Check sheet for the modelled part. Datum: model origin and axes. Units: mm. Face numbers are marked on the shaded views. Round coordinates to 2 decimals unless told otherwise and drop trailing zeros. Order: outer loops, then holes, each group sorted by start corner. A loop starts at its lowest first (then second) coordinate and runs counter-clockwise, first axis right, second up. Notation, with made-up numbers: (18, 80) -> (75, 80) arc R7 ccw to (75, 88) -> close; hole circle Ø8 at (33.5, 16). An arc over 180 degrees is marked (long way). Answer in a Markdown table with one row per item.
```python
from build123d import *

# Parameters (mm, degrees)
SKETCH1_W          = 76.2
SKETCH1_H          = 182.7422304
BASE_FLANGE1_DEPTH = 1.5875
CUT_EXTRUDE1_REACH = 199.999
SKETCH6_R          = 3.3782
SKETCH7_R          = 9.525
CUT_EXTRUDE2_DEPTH = 198.999199311
HEM1_START         = -182.7422304
HEM1_DEPTH         = 182.7422304
HEM1_2_DEPTH       = 182.7422304


# Read off the part's stored shape, not the designer's step: Hem1
# Sheet-metal steps are written as plain solids
with BuildPart() as part:
    # Sketch1 → Base-Flange1 (new body)
    with BuildSketch(Plane(origin=(0, 0, 0), x_dir=(1, 0, 0), z_dir=(0, 1, 0))):
        with Locations((-38.1, 91.3711152)):
            Rectangle(SKETCH1_W, SKETCH1_H)
    extrude(amount=-BASE_FLANGE1_DEPTH)

    # Sketch6 → Cut-Extrude1 (cut, up to next)
    with BuildSketch(Plane(origin=(0, 0, 0), x_dir=(1, 0, 0), z_dir=(0, 1, 0)), mode=Mode.PRIVATE) as cut_extrude1_sk1:
        with Locations(Location((-57.15, 170.0422304, 0), (0, 0, 270))):
            Circle(SKETCH6_R)
    cut_extrude1_tool1 = extrude(cut_extrude1_sk1.sketch, amount=-CUT_EXTRUDE1_REACH, mode=Mode.PRIVATE) & part.part
    # Sketch6 → Cut-Extrude1 (cut, up to next)
    with BuildSketch(Plane(origin=(0, 0, 0), x_dir=(1, 0, 0), z_dir=(0, 1, 0)), mode=Mode.PRIVATE) as cut_extrude1_sk2:
        with Locations(Location((-19.05, 170.0422304, 0), (0, 0, 270))):
            Circle(SKETCH6_R)
    cut_extrude1_tool2 = extrude(cut_extrude1_sk2.sketch, amount=-CUT_EXTRUDE1_REACH, mode=Mode.PRIVATE) & part.part
    # Sketch6 → Cut-Extrude1 (cut, up to next)
    with BuildSketch(Plane(origin=(0, 0, 0), x_dir=(1, 0, 0), z_dir=(0, 1, 0)), mode=Mode.PRIVATE) as cut_extrude1_sk3:
        with Locations(Location((-19.05, 107.14228, 0), (0, 0, 270))):
            Circle(SKETCH6_R)
    cut_extrude1_tool3 = extrude(cut_extrude1_sk3.sketch, amount=-CUT_EXTRUDE1_REACH, mode=Mode.PRIVATE) & part.part
    # Sketch6 → Cut-Extrude1 (cut, up to next)
    with BuildSketch(Plane(origin=(0, 0, 0), x_dir=(1, 0, 0), z_dir=(0, 1, 0)), mode=Mode.PRIVATE) as cut_extrude1_sk4:
        with Locations(Location((-57.15, 107.14228, 0), (0, 0, 270))):
            Circle(SKETCH6_R)
    cut_extrude1_tool4 = extrude(cut_extrude1_sk4.sketch, amount=-CUT_EXTRUDE1_REACH, mode=Mode.PRIVATE) & part.part
    add(cut_extrude1_tool1.solids().sort_by_distance((-57.15, 0, -170.04223))[0], mode=Mode.SUBTRACT)
    add(cut_extrude1_tool2.solids().sort_by_distance((-19.05, 0, -170.04223))[0], mode=Mode.SUBTRACT)
    add(cut_extrude1_tool3.solids().sort_by_distance((-19.05, 0, -107.14228))[0], mode=Mode.SUBTRACT)
    add(cut_extrude1_tool4.solids().sort_by_distance((-57.15, 0, -107.14228))[0], mode=Mode.SUBTRACT)

    # Sketch7 → Cut-Extrude2 (cut, through all)
    with BuildSketch(Plane(origin=(0, 0, 0), x_dir=(1, 0, 0), z_dir=(0, 1, 0))):
        with Locations(Location((-38.1, 46.7957408, 0), (0, 0, 270))):
            Circle(SKETCH7_R)
    extrude(amount=-CUT_EXTRUDE2_DEPTH, mode=Mode.SUBTRACT)

    # Hem1 outline → Hem1 (cut)
    with BuildSketch(Plane.XY.offset(HEM1_START)):
        with BuildLine():
            ThreePointArc((-74.5625, -1.5875), (-75.70257264, -1.125432101), (-76.199236463, 0))
            Line((-76.199236463, 0), (-76.2, 0))
            Line((-76.2, 0), (-76.2, -1.5875))
            Line((-76.2, -1.5875), (-74.5625, -1.5875))
        make_face()
        with BuildLine():
            ThreePointArc((-0.000763537, 0), (-0.49742736, -1.125432101), (-1.6375, -1.5875))
            Line((-1.6375, -1.5875), (0, -1.5875))
            Line((0, -1.5875), (0, 0))
            Line((0, 0), (-0.000763537, 0))
        make_face()
    extrude(amount=HEM1_DEPTH, mode=Mode.SUBTRACT)

    # Hem1 2 outline → Hem1 2 (add)
    with BuildSketch(Plane.XY.offset(HEM1_START)):
        with BuildLine():
            Line((-66.675, 0.1), (-66.675, 1.6875))
            Line((-66.675, 1.6875), (-74.5625, 1.6875))
            ThreePointArc((-74.5625, 1.6875), (-75.737932101, 1.19007264), (-76.199236463, 0))
            Line((-76.199236463, 0), (-74.5625, 0))
            ThreePointArc((-74.5625, 0), (-74.6125, 0.05), (-74.5625, 0.1))
            Line((-74.5625, 0.1), (-66.675, 0.1))
        make_face()
        with BuildLine():
            ThreePointArc((-1.6375, 0.1), (-1.5875, 0.05), (-1.6375, 0))
            Line((-1.6375, 0), (-0.000763537, 0))
            ThreePointArc((-0.000763537, 0), (-0.462067899, 1.19007264), (-1.6375, 1.6875))
            Line((-1.6375, 1.6875), (-9.525, 1.6875))
            Line((-9.525, 1.6875), (-9.525, 0.1))
            Line((-9.525, 0.1), (-1.6375, 0.1))
        make_face()
    extrude(amount=HEM1_2_DEPTH)


solid = part.part
```
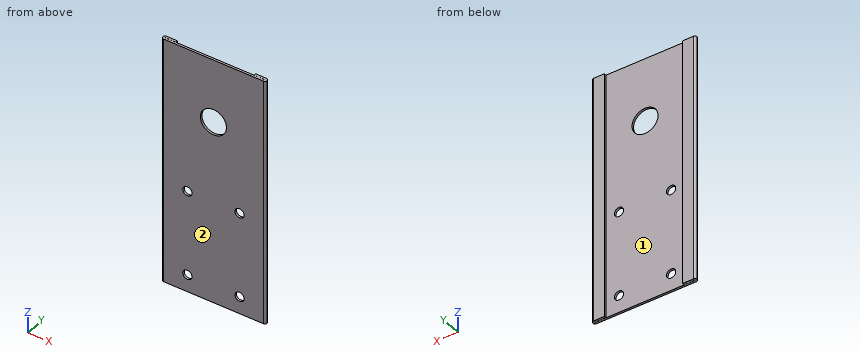
(1) Section check C-C on x = -19.05. Record the boundary of the cut face in (y, z), plus the area to 3 significant figures.
Solutions:
| item | result |
|---|---|
| outline | (-1.59, -182.74) -> (0, -182.74) -> (0, -173.42) -> (-1.59, -173.42) -> close; (-1.59, -166.66) -> (0, -166.66) -> (0, -110.52) -> (-1.59, -110.52) -> close; (-1.59, -103.76) -> (0, -103.76) -> (0, 0) -> (-1.59, 0) -> close |
| area | 269 mm^2 |
(2) Draft check along X on the marked faces 1 and 2. Enter one of: pulls with the +X half, pulls with the -X half, needs draft (parallel to the pull), parting line crosses it, or undercut.
Solutions:
| item | result |
|---|---|
| face 1 | undercut |
| face 2 | needs draft |
(3) Section check A-A on x = -38.1. Record the boundary of the cut face in (y, z), plus the area to 3 significant figures.
Solutions:
| item | result |
|---|---|
| outline | (-1.59, -182.74) -> (0, -182.74) -> (0, -56.32) -> (-1.59, -56.32) -> close; (-1.59, -37.27) -> (0, -37.27) -> (0, 0) -> (-1.59, 0) -> close |
| area | 260 mm^2 |
(4) Depth check by flat-ended pin: pin 1 Ø5.5 at (x, z) = (-57.15, -170.04) entering from +Y; pin 2 Ø5 at (x, z) = (-40.5, -118.5) entering from +Y; pin 3 Ø0.5 at (y, z) = (1, -47.5) entering from -X; pin 4 Ø1.7 at (y, z) = (1, -80.5) entering from +X. Enter the tip coordinate at first touch or a pass-through.
Solutions:
| item | result |
|---|---|
| pin 1 | through |
| pin 2 | y = 0 |
| pin 3 | x = -76.04 |
| pin 4 | x = 0 |
(5) Section check B-B on y = 0.8. Record the boundary of the cut face in (x, z) (3 decimals).
Solutions:
| item | result |
|---|---|
| outline | (-76.018, -182.742) -> (-66.675, -182.742) -> (-66.675, 0) -> (-76.018, 0) -> close; (-9.525, -182.742) -> (-0.182, -182.742) -> (-0.182, 0) -> (-9.525, 0) -> close |
(6) Scan lines: probe 1 along X at (y, z) = (0.15, -23.5) (3 decimals); probe 2 along Y at (x, z) = (-45, -80.5); probe 3 along Z at (x, y) = (-54.5, -1.1). Record each from-to range of solid material in increasing order. Write a range as from..to.
Solutions:
| item | result |
|---|---|
| probe 1 | -76.197..-66.675, -9.525..-0.003 |
| probe 2 | -1.59..0 |
| probe 3 | -182.74..-172.14, -167.95..-109.24, -105.05..0 |
